from build123d import *

# Parameters (mm, degrees)
BOSS_EXTRUDE1_DEPTH = 63.5
SKETCH2_W           = 50.8
SKETCH2_H           = 12.7
CUT_EXTRUDE2_DEPTH  = 39.1


with BuildPart() as part:
    # Sketch1 → Boss-Extrude1 (new body)
    with BuildSketch(Plane.XY):
        Polygon((19.05, 0), (-19.05, 0), (-19.05, 50.8), align=None)
    extrude(amount=BOSS_EXTRUDE1_DEPTH)

    # Sketch2 → Cut-Extrude2 (cut, through all)
    with BuildSketch(Plane.ZY.offset(19.05)):
        with Locations((31.75, 44.45)):
            Rectangle(SKETCH2_W, SKETCH2_H)
    extrude(amount=-CUT_EXTRUDE2_DEPTH, mode=Mode.SUBTRACT)


solid = part.part
Design review of the part built by this model. Coordinates are the model's own, in mm. A direction names the side the tool comes from. Coordinates: 2 decimals unless noted, no trailing zeros. Loops run counter-clockwise (first coordinate to the right, second up) from the corner with the lowest first, then second, coordinate; pieces in that order, holes last. Notation, with made-up numbers: M -28,-34.5 L 5,-34.5 A28 cw 5,-12.5 Z; hole C -18,39 d11. An arc over 180 degrees is marked long. Use one line per item in the form item = value.
(1) Consider section D-D (z = 24). Write out the cut boundary in (x, y) (3 decimals).
Return value:
outline = M -19.05,0 L 19.05,0 L -9.525,38.1 L -19.05,38.1 Z
(2) Clearance check with a flat-ended pin moving along its axis: P1, Ø5, axis at x = -16, z = 34.5, coming from the +Y side. State where the tip first meets the part, or that it passes through.
Return value:
P1 = 38.1
(3) Consider section A-A (y = 47). Write out the cut boundary in (x, z).
Return value:
outline = M -19.05,0 L -16.2,0 L -16.2,6.35 L -19.05,6.35 Z; M -19.05,57.15 L -16.2,57.15 L -16.2,63.5 L -19.05,63.5 Z
(4) For faces 5 (the face through (-15, 43, 57.15)), 6 (the face through (0, 0, 31)), list the 3-axis set-ups (+Z, -Z, +X, -X, +Y, -Y) from which the entire face can be reached by the end or side of a thin tool; tool diameter is ignored.
Return value:
face_5 = +X, -X, +Y
face_6 = +Z, -Z, +X, -X, -Y
(5) Consider section C-C (y = 16). Write out the cut boundary in (x, z).
Return value:
outline = M -19.05,0 L 7.05,0 L 7.05,63.5 L -19.05,63.5 Z
(6) Draft analysis for pull direction Z (two halves, no side actions). For faces 1 (the face through (-14, 38.1, 31)), 2 (the face through (-19.05, 19, 31)), 3 (the face through (-8, 14, 0)), 4 (the face through (-8, 14, 63.5)), state which applies: pulls with the +Z half, pulls with the -Z half, needs draft (parallel to the pull), parting line crosses it, or undercut.
Return value:
face_1 = undercut
face_2 = needs draft
face_3 = pulls with the -Z half
face_4 = pulls with the +Z half
(7) Consider section B-B (x = -16). Write out the cut boundary in (y, z), and give its area (3 significant figures).
Return value:
outline = M 0,0 L 46.73,0 L 46.73,6.35 L 38.1,6.35 L 38.1,57.15 L 46.73,57.15 L 46.73,63.5 L 0,63.5 Z
area = 2,530 mm2
(8) For line 1 along Z through (x, y) = (-15, 41); line 2 along Y through (x, z) = (-10, 54); line 3 along Y through (x, z) = (6.5, 9.5), list the stretches that pass through material, from the lowest coordinate up. Write a range as from..to.
Return value:
line_1 = 0..6.35, 57.15..63.5
line_2 = 0..38.1
line_3 = 0..16.73
